Can you work these out from the drawing? Everything is in mm from the part's minimum corner. Give positions to 0.01 mm unless a question says otherwise; leave off trailing zeros. Loops run counter-clockwise (first coordinate to the right, second up) from the corner with the lowest first, then second, coordinate; pieces in that order, holes last.
Q1. If we section it at B-B (x = 39): Please give me the cut outline in (y, z).
Q2. We'd pull the mould along Z, two halves only. Please class the marked faces 1, 2, 3 and 4: +Z half, -Z half, draft (parallel to the pull), parting line (faces both ways), or undercut.
Q3. If we section it at C-C (y = 9): Please give me the cut outline in (x, z), plus the area to 3 significant figures.
Q4. If we section it at A-A (z = 12.7): Please give me the cut outline in (x, y).
Q5. I need wall thicknesses on line 1 (X direction, y = 1.75, z = 13) (1 decimal); line 2 (Z direction, x = 41, y = 5.5) (1 decimal); line 3 (X direction, y = 6.25, z = 13.25) (1 decimal). Which ranges of each line are inside material? Lowest first, please.
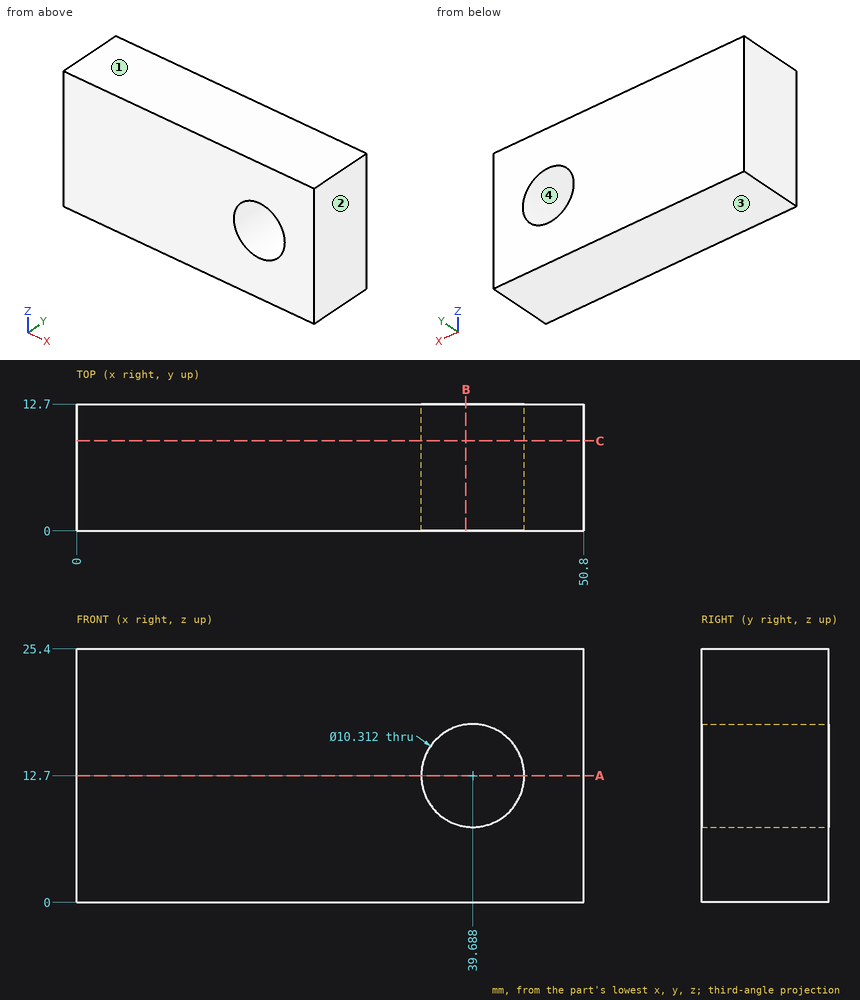
Check sheet entries:
1. outline: (0, 0) - (12.7, 0) - (12.7, 7.59) - (0, 7.59) - close; (0, 17.81) - (12.7, 17.81) - (12.7, 25.4) - (0, 25.4) - close
2. face 1: +Z half
2. face 2: draft
2. face 3: -Z half
2. face 4: undercut
3. outline: (0, 0) - (50.8, 0) - (50.8, 25.4) - (0, 25.4) - close; hole circle Ø10.31 at (39.69, 12.7)
3. area: 1,210 mm2
4. outline: (0, 0) - (34.53, 0) - (34.53, 12.7) - (0, 12.7) - close; (44.84, 0) - (50.8, 0) - (50.8, 12.7) - (44.84, 12.7) - close
5. line 1: x = 0 to 34.5, 44.8 to 50.8
5. line 2: z = 0 to 7.7, 17.7 to 25.4
5. line 3: x = 0 to 34.6, 44.8 to 50.8
